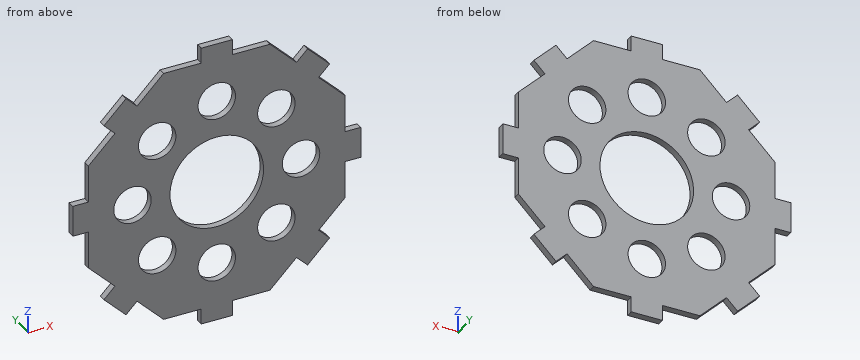
from build123d import *

# Parameters (mm, degrees)
SKETCH1_R           = 6
SKETCH1_R_2         = 15
BOSS_EXTRUDE1_DEPTH = 2.2


with BuildPart() as part:
    # Sketch1 → Boss-Extrude1 (new body)
    with BuildSketch(Plane(origin=(0, 0, 0), x_dir=(1, 0, 0), z_dir=(0, 1, 0))):
        Polygon((-55.857081241, 81.871122291), (-55.857081241, 86.871122291), (-65.857081241, 86.871122291), (-65.857081241, 81.871122291), (-77.894941, 81.871122291), (-86.406993267, 73.359070024), (-89.942527173, 76.89460393), (-97.013594985, 69.823536118), (-93.478061079, 66.288002212), (-101.990113346, 57.775949945), (-101.990113346, 45.738090186), (-106.990113346, 45.738090186), (-106.990113346, 35.738090186), (-101.990113346, 35.738090186), (-101.990113346, 23.700230426), (-93.478061079, 15.188178159), (-97.013594985, 11.652644253), (-89.942527173, 4.581576441), (-86.406993267, 8.117110347), (-77.894941, -0.39494192), (-65.857081241, -0.39494192), (-65.857081241, -5.39494192), (-55.857081241, -5.39494192), (-55.857081241, -0.39494192), (-43.819221481, -0.39494192), (-35.307169214, 8.117110347), (-31.771635308, 4.581576441), (-24.700567496, 11.652644253), (-28.236101402, 15.188178159), (-19.724049135, 23.700230426), (-19.724049135, 35.738090186), (-14.724049135, 35.738090186), (-14.724049135, 45.738090186), (-19.724049135, 45.738090186), (-19.724049135, 57.775949945), (-28.236101402, 66.288002212), (-24.700567496, 69.823536118), (-31.771635308, 76.89460393), (-35.307169214, 73.359070024), (-43.819221481, 81.871122291), align=None)
        with Locations(Location((-60.857081241, 67.738090186, 0), (0, 0, 270))):
            Circle(SKETCH1_R, mode=Mode.SUBTRACT)
        with Locations(Location((-41.765198148, 59.829973278, 0), (0, 0, 270))):
            Circle(SKETCH1_R, mode=Mode.SUBTRACT)
        with Locations(Location((-33.857081241, 40.738090186, 0), (0, 0, 270))):
            Circle(SKETCH1_R, mode=Mode.SUBTRACT)
        with Locations(Location((-41.765198148, 21.646207094, 0), (0, 0, 270))):
            Circle(SKETCH1_R, mode=Mode.SUBTRACT)
        with Locations(Location((-60.857081241, 13.738090186, 0), (0, 0, 270))):
            Circle(SKETCH1_R, mode=Mode.SUBTRACT)
        with Locations(Location((-79.948964333, 21.646207094, 0), (0, 0, 270))):
            Circle(SKETCH1_R, mode=Mode.SUBTRACT)
        with Locations(Location((-87.857081241, 40.738090186, 0), (0, 0, 270))):
            Circle(SKETCH1_R, mode=Mode.SUBTRACT)
        with Locations(Location((-79.948964333, 59.829973278, 0), (0, 0, 270))):
            Circle(SKETCH1_R, mode=Mode.SUBTRACT)
        with Locations(Location((-60.857081241, 40.738090186, 0), (0, 0, 270))):
            Circle(SKETCH1_R_2, mode=Mode.SUBTRACT)
    extrude(amount=BOSS_EXTRUDE1_DEPTH)


solid = part.part
Geometry check sheet. Reference: the model listing, model coordinates, mm. Coordinates: 2 decimals unless noted, no trailing zeros. Order: outer loops, then holes, each group sorted by start corner. A loop starts at its lowest first (then second) coordinate and runs counter-clockwise, first axis right, second up. Notation, with made-up numbers: (4, 7) - (29, 7) arc R18 cw to (29, 23) - close; hole circle Ø1 at (25.5, 56.5). An arc over 180 degrees is marked (long way). Answer in a Markdown table with one row per item. Add a question column.
1) Cross-section at B-B, the plane z = -44.5. Record the cut outline in (x, y).
2) Cross-section at D-D, the plane x = -98.5. Record the cut outline in (y, z), then the cut area to 3 significant figures.
3) Cross-section at C-C, the plane z = -22.5. Record the cut outline in (x, y), then the cut area to 3 significant figures.
4) Gauge pin test, flat ends, axial feed: P1, Ø1.1, axis at x = -69.5, y = 0.5, coming from the -Z side; P2, Ø0.7, axis at x = -73, y = 1.5, coming from the +Z side; P3, Ø19, axis at x = -41.77, z = -59.83, coming from the -Y side; P4, Ø1.1, axis at y = 1, z = -28, coming from the -X side. Record the tip position at first contact, or that the pin passes through.
5) Material ranges on line 1 along Z through (x, y) = (-61, 1.1); line 2 along Z through (x, y) = (-25, 1); line 3 along X through (y, z) = (0.35, -25), recorded low to high. Write a range as [from, to].
6) Cross-section at A-A, the plane x = -26. Record the cut outline in (y, z), then the cut area to 3 significant figures.
Check result:
| question | item | result |
|---|---|---|
| 1 | outline | (-106.99, 0) - (-92.53, 0) - (-92.53, 2.2) - (-106.99, 2.2) - close; (-83.18, 0) - (-75.38, 0) - (-75.38, 2.2) - (-83.18, 2.2) - close; (-46.34, 0) - (-38.53, 0) - (-38.53, 2.2) - (-46.34, 2.2) - close; (-29.18, 0) - (-14.72, 0) - (-14.72, 2.2) - (-29.18, 2.2) - close |
| 2 | outline | (0, -61.27) - (2.2, -61.27) - (2.2, -20.21) - (0, -20.21) - close |
| 2 | area | 90.3 mm² |
| 3 | outline | (-100.79, 0) - (-85.89, 0) - (-85.89, 2.2) - (-100.79, 2.2) - close; (-74.01, 0) - (-47.7, 0) - (-47.7, 2.2) - (-74.01, 2.2) - close; (-35.83, 0) - (-20.92, 0) - (-20.92, 2.2) - (-35.83, 2.2) - close |
| 3 | area | 123 mm² |
| 4 | P1 | stops at z = -81.87 |
| 4 | P2 | stops at z = 0.39 |
| 4 | P3 | stops at y = 0 |
| 4 | P4 | stops at x = -101.99 |
| 5 | line 1 | z = [-86.87, -73.74], [-61.74, -55.74], [-25.74, -19.74], [-7.74, 5.39] |
| 5 | line 2 | z = [-70.12, -69.52], [-63.05, -18.42], [-11.95, -11.35] |
| 5 | line 3 | x = [-101.99, -84.92], [-74.97, -46.74], [-36.79, -19.72] |
| 6 | outline | (0, -71.12) - (2.2, -71.12) - (2.2, -68.52) - (0, -68.52) - close; (0, -64.05) - (2.2, -64.05) - (2.2, -17.42) - (0, -17.42) - close; (0, -12.95) - (2.2, -12.95) - (2.2, -10.35) - (0, -10.35) - close |
| 6 | area | 114 mm² |
